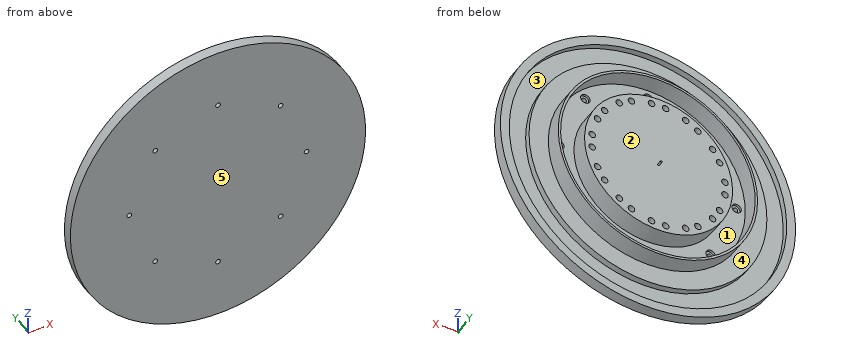
from build123d import *

# Parameters (mm, degrees)
SKETCH6_R           = 10
CUT_EXTRUDE2_DEPTH  = 5
SKETCH7_R           = 5
CUT_EXTRUDE3_DEPTH  = 447.09219899
SKETCH8_R           = 157.5
BOSS_EXTRUDE1_DEPTH = 40
SKETCH9_R           = 7
CUT_EXTRUDE4_DEPTH  = 35
CIRPATTERN1_COUNT   = 12
SKETCH10_R          = 2.000359625
BOSS_EXTRUDE2_DEPTH = 10


with BuildPart() as part:
    # Sketch3 → Revolve1 (revolve)
    with BuildSketch(Plane(origin=(0, 0, 0), x_dir=(0, 0, -1), z_dir=(1, 0, 0))):
        Polygon((-212, 8.070339729), (-212, 45.570339729), (-207, 45.570339729), (-207, 8.070339729), (-0.848831398, 8.070339729), (-0.848831398, 11.780945064), (0, 11.780945064), (0, 8.070339729), (0, -14.429660271), (-314, -14.429660271), (-314, 8.070339729), (-295, 8.070339729), (-295, -4.929660271), (-253, -4.929660271), (-253, 8.070339729), align=None)
    revolve(axis=Axis((0, 120.738006406, 0), (0, -1, 0)))

    # Sketch6 → Cut-Extrude2 (cut)
    with BuildSketch(Plane(origin=(0, 8.070339729, 0), x_dir=(1, 0, 0), z_dir=(0, 1, 0))):
        with Locations(Location((-133.289628254, 133.289628254, 0), (0, 0, 270))):
            Circle(SKETCH6_R)
        with Locations(Location((133.289628254, 133.289628254, 0), (0, 0, 270))):
            Circle(SKETCH6_R)
        with Locations(Location((-133.289628254, -133.289628254, 0), (0, 0, 90))):
            Circle(SKETCH6_R)
        with Locations(Location((133.289628254, -133.289628254, 0), (0, 0, 90))):
            Circle(SKETCH6_R)
        with Locations(Location((0, 188.5, 0), (0, 0, 270))):
            Circle(SKETCH6_R)
        with Locations(Location((188.5, 0, 0), (0, 0, 270))):
            Circle(SKETCH6_R)
        with Locations(Location((0, -188.5, 0), (0, 0, 90))):
            Circle(SKETCH6_R)
        with Locations(Location((-188.5, 0, 0), (0, 0, 90))):
            Circle(SKETCH6_R)
    extrude(amount=-CUT_EXTRUDE2_DEPTH, mode=Mode.SUBTRACT)

    # Sketch7 → Cut-Extrude3 (cut, through all)
    with BuildSketch(Plane(origin=(0, 3.070339729, 0), x_dir=(1, 0, 0), z_dir=(0, 1, 0))):
        with Locations(Location((0, 188.5, 0), (0, 0, 270))):
            Circle(SKETCH7_R)
        with Locations(Location((133.289628254, 133.289628254, 0), (0, 0, 270))):
            Circle(SKETCH7_R)
        with Locations(Location((-133.289628254, 133.289628254, 0), (0, 0, 90))):
            Circle(SKETCH7_R)
        with Locations(Location((188.5, 0, 0), (0, 0, 90))):
            Circle(SKETCH7_R)
        with Locations(Location((133.289628254, -133.289628254, 0), (0, 0, 90))):
            Circle(SKETCH7_R)
        with Locations(Location((0, -188.5, 0), (0, 0, 90))):
            Circle(SKETCH7_R)
        with Locations(Location((-188.5, 0, 0), (0, 0, 270))):
            Circle(SKETCH7_R)
        with Locations(Location((-133.289628254, -133.289628254, 0), (0, 0, 270))):
            Circle(SKETCH7_R)
    extrude(amount=-CUT_EXTRUDE3_DEPTH, mode=Mode.SUBTRACT)

    # Sketch8 → Boss-Extrude1 (add)
    with BuildSketch(Plane(origin=(0, 8.070339729, 0), x_dir=(1, 0, 0), z_dir=(0, 1, 0))):
        with Locations(Location((0, 0, 0), (0, 0, 270))):
            Circle(SKETCH8_R)
    extrude(amount=BOSS_EXTRUDE1_DEPTH)

    # Sketch9 → Cut-Extrude4 (cut)
    with BuildSketch(Plane(origin=(0, 48.070339729, 0), x_dir=(1, 0, 0), z_dir=(0, 1, 0))):
        with Locations(Location((-15, 141.25, 0), (0, 0, 270))):
            Circle(SKETCH9_R)
        with Locations(Location((15, 141.25, 0), (0, 0, 270))):
            Circle(SKETCH9_R)
    cut_extrude4 = extrude(amount=-CUT_EXTRUDE4_DEPTH, mode=Mode.SUBTRACT)

    # CirPattern1: Cut-Extrude4 ×12 about axis
    cirpattern1_axis = Axis((0, 0, 0), (0, 1, 0))
    for i in range(1, CIRPATTERN1_COUNT):
        add(cut_extrude4.rotate(cirpattern1_axis, i * 360 / CIRPATTERN1_COUNT), mode=Mode.SUBTRACT)

    # Sketch10 → Boss-Extrude2 (add)
    with BuildSketch(Plane(origin=(0, 48.070339729, 0), x_dir=(1, 0, 0), z_dir=(0, 1, 0))):
        with Locations(Location((0, 0, 0), (0, 0, 270))):
            Circle(SKETCH10_R)
    extrude(amount=BOSS_EXTRUDE2_DEPTH)


solid = part.part
Could you check a few things on this model? Use its own coordinates, in mm. Face numbers are marked on the shaded views. A direction names the side the tool comes from. Coordinates: 2 decimals unless noted, no trailing zeros. Write each loop counter-clockwise with the first axis right and the second up, starting at its lowest first coordinate (ties: lowest second). Pieces come first, ordered by that corner, then holes. Notation, with made-up numbers: (40, 19) - (51, 19) arc R29 cw to (51, 56) - close; hole circle Ø2 at (-26, 13). An arc over 180 degrees is marked (long way). Write item = value, one per line.
1) Will these pins go through, and if not, where does the flat tip stop? pin 1 Ø1.5 at (y, z) = (-4.5, -90) entering from -X; pin 2 Ø2 at (y, z) = (1.5, 186) entering from +X; pin 3 Ø1.5 at (x, y) = (83.5, 13) entering from -Z.
Result set:
pin_1 = -301.05
pin_2 = 253.71
pin_3 = -195.18
2) Please list where these lines run through material, in increasing order: line 1 (X direction, y = 0.5, z = -7); line 2 (X direction, y = -1, z = 71.5); line 3 (Z direction, x = 42.5, y = 43). Write a range as [from, to].
Result set:
line_1 = [-313.92, -294.92], [-252.9, 252.9], [294.92, 313.92]
line_2 = [-305.75, -286.2], [-242.69, 242.69], [286.2, 305.75]
line_3 = [-207.7, -202.59], [-151.66, 151.66], [202.59, 207.7]
3) Suppose I cut it at C-C on x = 265.5. Please give me the cut outline in (y, z), plus the area to 3 significant figures.
Result set:
outline = (-14.43, -167.65) - (8.07, -167.65) - (8.07, -128.59) - (-4.93, -128.59) - (-4.93, 128.59) - (8.07, 128.59) - (8.07, 167.65) - (-14.43, 167.65) - close
area = 4,200 mm2
4) Suppose I cut it at A-A on y = 24. State how many separate pieces and enclosed holes the cut face has, plus the area to 3 significant figures.
Result set:
separate_pieces = 2
enclosed_holes = 25
area = 80,800 mm2
5) Suppose I cut it at B-B on z = -268. Please give me the cut outline in (x, y), plus the area to 3 significant figures.
Result set:
outline = (-163.62, -14.43) - (163.62, -14.43) - (163.62, 8.07) - (123.29, 8.07) - (123.29, -4.93) - (-123.29, -4.93) - (-123.29, 8.07) - (-163.62, 8.07) - close
area = 4,160 mm2
6) For the marked faces 4 and 5, which set-ups out of +Z, -Z, +X, -X, +Y, -Y let a thin tool reach every point of the face, with its end or its side?
Result set:
face_4 = +Y
face_5 = +Z, -Z, +X, -X, -Y
7) We'd pull the mould along X, two halves only. Please class the marked faces 1, 2 and 3: +X half, -X half, draft (parallel to the pull), parting line (faces both ways), or undercut.
Result set:
face_1 = undercut
face_2 = draft
face_3 = undercut
8) Suppose I cut it at D-D on z = 243.5. Please give me the cut outline in (x, y), plus the area to 3 significant figures.
Result set:
outline = (-198.25, -14.43) - (198.25, -14.43) - (198.25, 8.07) - (166.53, 8.07) - (166.53, -4.93) - (68.68, -4.93) - (68.68, 8.07) - (-68.68, 8.07) - (-68.68, -4.93) - (-166.53, -4.93) - (-166.53, 8.07) - (-198.25, 8.07) - close
area = 6,380 mm2
